CAD build for the part. Positions are in the model's coordinates, mm. Face numbers are marked on the shaded views. A direction names the side the tool comes from. Round coordinates to 2 decimals unless told otherwise and drop trailing zeros. Write each loop counter-clockwise with the first axis right and the second up, starting at its lowest first coordinate (ties: lowest second). Pieces come first, ordered by that corner, then holes. Notation, with made-up numbers: M 21.25,52 L 38.25,52 A23 cw 38.25,81 Z; hole C 64,-18.75 d7. An arc over 180 degrees is marked long. Write each question's results on one line, items separated by ' | '. Start each with the question number.
```python
from build123d import *

# Parameters (mm, degrees)
F0_W      = 28
F0_H      = 40
F1_DEPTH  = 10
F2_W      = 4
F2_H      = 10
F2_W_2    = 17
F2_H_2    = 8.5
F3_DEPTH  = 32
F5_DEPTH  = 24.001
F6_W      = 28
F6_H      = 8
F7_DEPTH  = 5
F8_R      = 1
F9_DEPTH  = 10.001
F10_R     = 2.25
F11_DEPTH = 9
F13_DEPTH = 10.001
F14_R     = 3.5


with BuildPart() as f1:
    # F0 (on Front) → F1 (new body)
    with BuildSketch(Plane.XZ):
        with Locations((0, 20)):
            Rectangle(F0_W, F0_H)
    extrude(amount=F1_DEPTH)

    # F2 (on face) → F3 (cut)
    with BuildSketch(Plane.XY.offset(40)):
        with Locations((-12, -5)):
            Rectangle(F2_W, F2_H)
        with Locations((12, -5)):
            Rectangle(F2_W, F2_H)
        with Locations((0, -5.75)):
            Rectangle(F2_W_2, F2_H_2)
    extrude(amount=-F3_DEPTH, mode=Mode.SUBTRACT)

    # F4 (on face) → F5 (cut, through all)
    with BuildSketch(Plane(origin=(-10, 0, 0), x_dir=(0, -1, 0), z_dir=(-1, 0, 0))):
        Polygon((1.5, 40), (10, 8), (10, 40), align=None)
    extrude(amount=-F5_DEPTH, mode=Mode.SUBTRACT)

    # F6 (on face) → F7 (join)
    with BuildSketch(Plane(origin=(0, 0, 0), x_dir=(-1, 0, 0), z_dir=(0, 1, 0))):
        with Locations((0, 4)):
            Rectangle(F6_W, F6_H)
    extrude(amount=F7_DEPTH)

    # F8 (on face) → F9 (cut, through all)
    with BuildSketch(Plane(origin=(0, 0, 0), x_dir=(-1, 0, 0), z_dir=(0, 1, 0))):
        with Locations((0, 30)):
            Circle(F8_R)
    extrude(amount=-F9_DEPTH, mode=Mode.SUBTRACT)

    # F10 (on face) → F11 (cut)
    with BuildSketch(Plane(origin=(0, 0, 0), x_dir=(1, 0, 0), z_dir=(0, 0, -1))):
        Circle(F10_R)
    extrude(amount=-F11_DEPTH, mode=Mode.SUBTRACT)

    # F12 (on face) → F13 (cut, through all)
    with BuildSketch(Plane(origin=(0, 0, 0), x_dir=(-1, 0, 0), z_dir=(0, 1, 0))):
        with BuildLine():
            Line((-2.25, 10), (-2.25, 8))
            Line((-2.25, 8), (2.25, 8))
            Line((2.25, 8), (2.25, 10))
            ThreePointArc((2.25, 10), (0, 12.25), (-2.25, 10))
        make_face()
    extrude(amount=-F13_DEPTH, mode=Mode.SUBTRACT)

    # F14
    f14_edges = [f1.edges().sort_by_distance(p)[0] for p in [
        (10, -5, 8),
        (-10, -5, 8),
    ]]
    fillet(f14_edges, radius=F14_R)


solid = f1.part
```
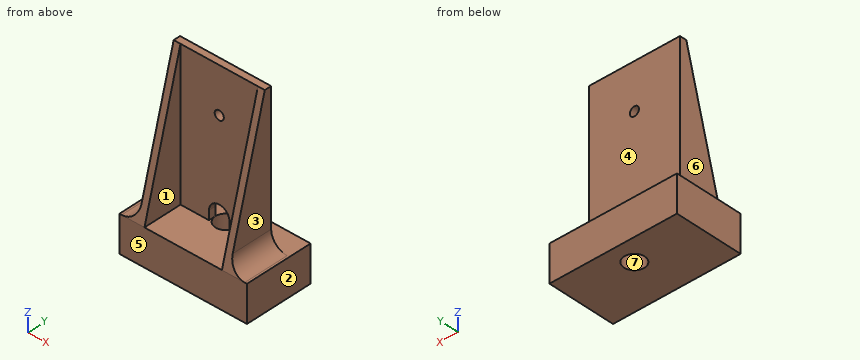
1) Wall check: line 1 along Y through (x, z) = (0, 5.5); line 2 along Z through (x, y) = (0, -0.4); line 3 along X through (y, z) = (-2, 19.5). Give the ranges that are in metal, low to high. Write a range as from..to.
2) Saw through at B-B, the plane x = 0. Write the cut outline in (y, z), plus the area to 3 significant figures.
3) Saw through at D-D, the plane z = 30. Write the cut outline in (x, y).
4) Saw through at A-A, the plane z = 4. Write the cut outline in (x, y), plus the area to 3 significant figures.
5) Pull direction X, two halves, no side cores. Call the marked faces 5, 6 and 7: pulls with the +X half, pulls with the -X half, needs draft (parallel to the pull), parting line crosses it, or undercut.
6) Drop flat-ended pins along their axis: pin 1 Ø4.5 at (y, z) = (-4, 17.5) entering from +X; pin 2 Ø1.5 at (x, z) = (2.5, 33.5) entering from +Y; pin 3 Ø4.5 at (y, z) = (-6, 23) entering from -X; pin 4 Ø7 at (x, y) = (0, 0) entering from -Z. Give the stop position or say it passes through.
7) Saw through at C-C, the plane y = 1.5. Write the cut outline in (x, z).
8) 3-axis set-ups, long thin cutter, end or side, ignore diameter. For the marked faces 1, 2, 3 and 4: which of +Z, -Z, +X, -X, +Y, -Y reach the whole face in a straight line?
Filled sheet:
1) line 1: y = -10..-2.25, 2.25..5 | line 2: z = 12.25..29, 31..40 | line 3: x = -10..-8.5, 8.5..10
2) outline: M -10,0 L -2.25,0 L -2.25,8 L -10,8 Z; M -1.5,12.25 L 0,12.25 L 0,29 L -1.5,29 Z; M -1.5,31 L 0,31 L 0,40 L -1.5,40 Z; M 2.25,0 L 5,0 L 5,8 L 2.25,8 Z | area: 123 mm^2
3) outline: M -10,-4.16 L -8.5,-4.16 L -8.5,-1.5 L -1,-1.5 L -1,0 L -10,0 Z; M 1,-1.5 L 8.5,-1.5 L 8.5,-4.16 L 10,-4.16 L 10,0 L 1,0 Z
4) outline: M -14,-10 L 14,-10 L 14,5 L -14,5 Z; hole C 0,0 d4.5 | area: 404 mm^2
5) face 5: needs draft | face 6: pulls with the -X half | face 7: undercut
6) pin 1: stops at x = 10 | pin 2: stops at y = 0 | pin 3: stops at x = -10 | pin 4: stops at z = 0
7) outline: M -14,0 L -1.68,0 L -1.68,8 L -14,8 Z; M 1.68,0 L 14,0 L 14,8 L 1.68,8 Z
8) face 1: +Z, -Y | face 2: +Z, -Z, +X, +Y, -Y | face 3: +Z, +X, +Y, -Y | face 4: +Z, +X, -X, +Y
